For this review, take the finished solid that the model builds, in its own axes (mm). A direction names the side the tool comes from. Round coordinates to 2 decimals unless told otherwise and drop trailing zeros. Write each loop counter-clockwise with the first axis right and the second up, starting at its lowest first coordinate (ties: lowest second). Pieces come first, ordered by that corner, then holes. Notation, with made-up numbers: (-8, 71.25) -> (1, 71.25) arc R22 ccw to (1, 102.25) -> close; hole circle Ø5 at (42, 33). An arc over 180 degrees is marked (long way). Write item = value, one per line. Start each with the question number.
```python
from build123d import *

# Parameters (mm, degrees)
BOSS_EXTRUDE1_DEPTH = 863.6
SKETCH3_R           = 3.175
CUT_EXTRUDE1_DEPTH  = 863.6
SKETCH2_W           = 304.8
SKETCH2_H           = 12.7
BOSS_EXTRUDE5_DEPTH = 863.6
SKETCH5_W           = 76.2
SKETCH5_H           = 25.4
BOSS_EXTRUDE6_DEPTH = 0.0127
SKETCH6_W           = 12.7
SKETCH6_H           = 12.7
BOSS_EXTRUDE8_DEPTH = 12.7
CUT_EXTRUDE2_DEPTH  = 137.668


with BuildPart() as part:
    # Sketch1 → Boss-Extrude1 (new body)
    with BuildSketch(Plane.XY):
        Polygon((0, 0), (38.1, 0), (38.1, 114.3), (19.716081556, 95.916081556), (0, 76.2), align=None)
    extrude(amount=BOSS_EXTRUDE1_DEPTH)

    # Sketch3 → Cut-Extrude1 (cut)
    with BuildSketch(Plane.XY.offset(863.6)):
        with Locations((19.05, 63.5)):
            Circle(SKETCH3_R)
    extrude(amount=-CUT_EXTRUDE1_DEPTH, mode=Mode.SUBTRACT)

    # Sketch2 → Boss-Extrude5 (add)
    with BuildSketch(Plane(origin=(0, 0, 0), x_dir=(-1, 0, 0), z_dir=(0, 0, -1))):
        with Locations((152.4, 6.35)):
            Rectangle(SKETCH2_W, SKETCH2_H)
    extrude(amount=-BOSS_EXTRUDE5_DEPTH)

    # Sketch5 → Boss-Extrude6 (add)
    with BuildSketch(Plane(origin=(0, 12.7, 0), x_dir=(1, 0, 0), z_dir=(0, 1, 0))):
        with Locations((-152.4, -34.636758867)):
            Rectangle(SKETCH5_W, SKETCH5_H)
        with Locations((-152.4, -828.963241133)):
            Rectangle(SKETCH5_W, SKETCH5_H)
    extrude(amount=BOSS_EXTRUDE6_DEPTH)

    # Sketch6 → Boss-Extrude8 (add)
    with BuildSketch(Plane(origin=(38.1, 0, 0), x_dir=(0, 0, -1), z_dir=(1, 0, 0))):
        with Locations((-380.236111085, 68.484263382)):
            Rectangle(SKETCH6_W, SKETCH6_H)
        with Locations((-483.363888915, 68.484263382)):
            Rectangle(SKETCH6_W, SKETCH6_H)
    extrude(amount=BOSS_EXTRUDE8_DEPTH)

    # Sketch7 → Cut-Extrude2 (cut)
    with BuildSketch(Plane.XY.offset(489.713888915)):
        Polygon((44.45, 68.812070036), (48.222471195, 68.812070036), (48.222471195, 74.834263382), (40.668527222, 74.834263382), (40.668527222, 68.812070036), align=None)
    extrude(amount=-CUT_EXTRUDE2_DEPTH, mode=Mode.SUBTRACT)


solid = part.part
```
1. Machinability: for faces 1 (the flat face through (-131, 0, 426)), 2 (the flat face through (-153, 12.713, 829)), which of the approach directions +Z, -Z, +X, -X, +Y, -Y give a long, thin tool a straight path to every point of the face, cutting with its end or side? Answer none if there is none.
2. Clearance check with flat-ended pins moving along their axes: pin 1 Ø1 at (y, z) = (35.5, 542) entering from +X; pin 2 Ø12.5 at (x, z) = (-171.5, 38.5) entering from +Y; pin 3 Ø3 at (y, z) = (56.5, 429) entering from -X; pin 4 Ø14 at (x, z) = (44.5, 378.5) entering from -Y. State where each tip first meets the part, or that it passes through.
3. Wall thickness on L1, parallel to X at y = 63, z = 430; L2, parallel to Y at x = -24, z = 570.5; L3, parallel to X at y = 55, z = 148: over which ranges is each line inside the solid? List them lowest first. Write a range as from..to.
4. Consider section C-C, the plane y = 39. Give the boundary of the cut face in (x, z), then the cut area to 3 significant figures.
5. Consider section D-D, the plane y = 104. Give the boundary of the cut face in (x, z).
6. Consider section A-A, the plane z = 161.5. Give the boundary of the cut face in (x, y) (3 decimals).
Outcome:
q1.face_1 = +Z, -Z, +X, -X, -Y
q1.face_2 = +Z, -Z, -X, +Y
q2.pin_1 = 38.1
q2.pin_2 = 12.71
q2.pin_3 = 0
q2.pin_4 = 0
q3.L1 = 0..15.91, 22.19..38.1
q3.L2 = 0..12.7
q3.L3 = 0..38.1
q4.outline = (0, 0) -> (38.1, 0) -> (38.1, 863.6) -> (0, 863.6) -> close
q4.area = 32,900 mm2
q5.outline = (27.8, 0) -> (38.1, 0) -> (38.1, 863.6) -> (27.8, 863.6) -> close
q6.outline = (-304.8, 0) -> (38.1, 0) -> (38.1, 114.3) -> (0, 76.2) -> (0, 12.7) -> (-304.8, 12.7) -> close; hole circle Ø6.35 at (19.05, 63.5)
